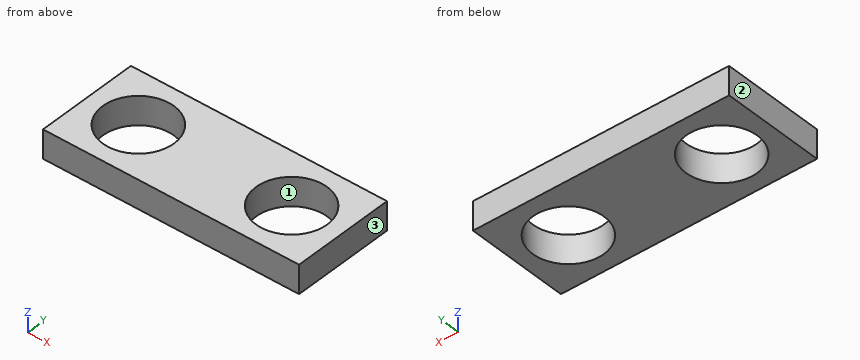
Autodesk Fusion 360 part; units mm, degrees
sketch "Sketch1" plane through (0, 0, 0) normal (0, 0, 1) x (1, 0, 0) in component "Component"
  line L0 (0, 0) -> (102.743, 0)
  line L1 (102.743, 0) -> (102.743, 41.2496)
  line L2 (102.743, 41.2496) -> (0, 41.2496)
  line L3 (0, 41.2496) -> (0, 0)
  dimension "d1" = 41.2496
  dimension "d10" = 102.743
extrude "Extrude1" add sketch "Sketch1" along normal blind 11.43 in component "Component"
sketch "Sketch2" plane through (0, 0, 11.43) normal (0, 0, 1) x (1, 0, 0) in component "Component"
  line L0 (0, 41.2496) -> (0, 0)
  line L1 (0, 0) -> (102.743, 0)
  line L2 (102.743, 0) -> (102.743, 41.2496)
  line L3 (102.743, 41.2496) -> (0, 41.2496)
  circle A0 centre (20.6248, 20.6248) radius 14.2748
  circle A1 centre (82.1182, 20.6248) radius 14.2748
  dimension "d4" = 28.5496
  dimension "d5" = 28.5496
  dimension "d6" = 20.6248
  dimension "d7" = 20.6248
  dimension "d8" = 20.6248
  dimension "d9" = 61.4934
extrude "Extrude2" cut sketch "Sketch2" against normal blind 11.43 contours A0 | A1 in component "Component"
component "Component" placed x (1, 0, 0) y (0, 1, 0) z (0, 0, 1) at (0, 0, 0)
Geometry check sheet. Reference: the model listing, model coordinates, mm. Face numbers are marked on the shaded views. Give positions to 0.01 mm unless a question says otherwise; leave off trailing zeros. Order: outer loops, then holes, each group sorted by start corner. A loop starts at its lowest first (then second) coordinate and runs counter-clockwise, first axis right, second up. Notation, with made-up numbers: (22.25, -22) - (36.25, -22) arc R27 ccw to (36.25, -5) - close; hole circle Ø5 at (57, 87.25). An arc over 180 degrees is marked (long way). Answer in a Markdown table with one row per item. Add a question column.
Q1. Material ranges on probe 1 along X at (y, z) = (17.5, 8.75); probe 2 along X at (y, z) = (17, 3.5); probe 3 along Y at (x, z) = (71, 5.5), recorded low to high. Write a range as from..to.
Q2. Mould release check, pull along X, two halves, no side actions. Record for the marked faces 1, 2 and 3: pulls with the +X half, pulls with the -X half, needs draft (parallel to the pull), parting line crosses it, or undercut.
Q3. Cross-section at A-A, the plane x = 14. Enter the section's corners in (y, z).
Q4. Cross-section at D-D, the plane y = 19.5. Enter the section's corners in (x, z), then the cut area to 3 significant figures.
Q5. Cross-section at B-B, the plane y = 13.5. Enter the section's corners in (x, z).
Q6. Cross-section at C-C, the plane z = 3. Enter the section's corners in (x, y).
Check values:
| question | item | result |
|---|---|---|
| 1 | probe 1 | x = 0..6.7, 34.55..68.19, 96.05..102.74 |
| 1 | probe 2 | x = 0..6.82, 34.43..68.31, 95.93..102.74 |
| 1 | probe 3 | y = 0..11.67, 29.58..41.25 |
| 2 | face 1 | undercut |
| 2 | face 2 | pulls with the -X half |
| 2 | face 3 | pulls with the +X half |
| 3 | outline | (0, 0) - (7.98, 0) - (7.98, 11.43) - (0, 11.43) - close; (33.27, 0) - (41.25, 0) - (41.25, 11.43) - (33.27, 11.43) - close |
| 4 | outline | (0, 0) - (6.39, 0) - (6.39, 11.43) - (0, 11.43) - close; (34.86, 0) - (67.89, 0) - (67.89, 11.43) - (34.86, 11.43) - close; (96.35, 0) - (102.74, 0) - (102.74, 11.43) - (96.35, 11.43) - close |
| 4 | area | 524 mm^2 |
| 5 | outline | (0, 0) - (8.26, 0) - (8.26, 11.43) - (0, 11.43) - close; (32.99, 0) - (69.75, 0) - (69.75, 11.43) - (32.99, 11.43) - close; (94.49, 0) - (102.74, 0) - (102.74, 11.43) - (94.49, 11.43) - close |
| 6 | outline | (0, 0) - (102.74, 0) - (102.74, 41.25) - (0, 41.25) - close; hole circle Ø28.55 at (20.62, 20.62); hole circle Ø28.55 at (82.12, 20.62) |
